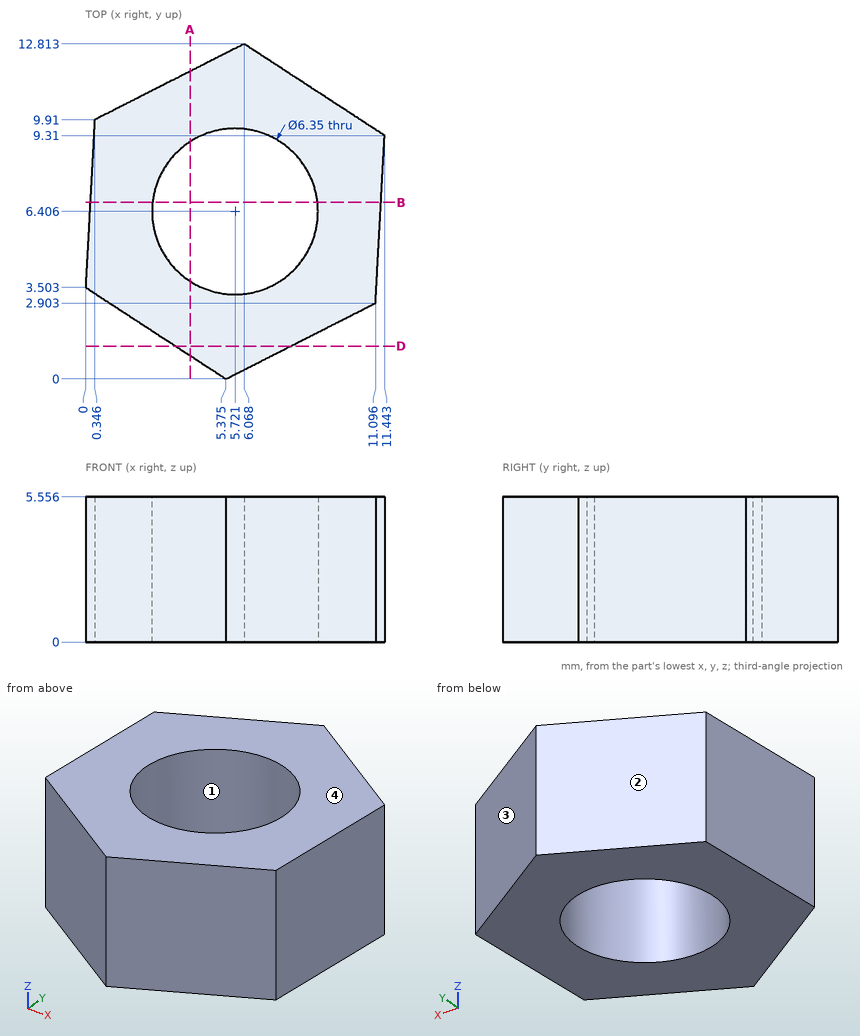
For this review, use the dimensioned drawing (mm, ordinates from the lowest corner) and the shaded views. Coordinates: 2 decimals unless noted, no trailing zeros. Write each loop counter-clockwise with the first axis right and the second up, starting at its lowest first coordinate (ties: lowest second). Pieces come first, ordered by that corner, then holes. Notation, with made-up numbers: (75.25, -31) - (89.25, -31) arc R18 ccw to (89.25, -25) - close; hole circle Ø11 at (-38, 75). An arc over 180 degrees is marked (long way). Answer in a Markdown table with one row per item. Add a question column.
Q1. Consider section A-A on x = 4. Give the boundary of the cut face in (y, z) (1 decimal).
Q2. Draft analysis for pull direction X (two halves, no side actions). For the marked faces 1, 2, 3 and 4, state which applies: +X half, -X half, draft (parallel to the pull), parting line (faces both ways), or undercut.
Q3. Consider section D-D on y = 1.25. Give the boundary of the cut face in (x, z).
Q4. Consider section B-B on y = 6.75. Give the boundary of the cut face in (x, z) (1 decimal).
Q5. Clearance check with flat-ended pins moving along their axes: pin 1 (1 mm diameter, centred on x = 7, z = 4, fed in from +Y); pin 2 (1 mm diameter, centred on x = 9.5, z = 4, fed in from +Y). State where each tip first meets the part, or that it passes through.
Q6. To check wall thickness, follow line 1 along Y through (x, z) = (6.75, 2.6); line 2 along Y through (x, z) = (4.75, 0.6) (1 decimal); line 3 along X through (y, z) = (6, 3.55) (1 decimal). State the ranges of each line that lie inside material, in increasing order. Write a range as from..to.
Answers below:
| question | item | result |
|---|---|---|
| 1 | outline | (0.9, 0) - (3.7, 0) - (3.7, 5.6) - (0.9, 5.6) - close; (9.1, 0) - (11.8, 0) - (11.8, 5.6) - (9.1, 5.6) - close |
| 2 | face 1 | undercut |
| 2 | face 2 | -X half |
| 2 | face 3 | +X half |
| 2 | face 4 | draft |
| 3 | outline | (3.46, 0) - (7.84, 0) - (7.84, 5.56) - (3.46, 5.56) - close |
| 4 | outline | (0.2, 0) - (2.6, 0) - (2.6, 5.6) - (0.2, 5.6) - close; (8.9, 0) - (11.3, 0) - (11.3, 5.6) - (8.9, 5.6) - close |
| 5 | pin 1 | y = 12.53 |
| 5 | pin 2 | y = 10.9 |
| 6 | line 1 | 0.7..3.4, 9.41..12.37 |
| 6 | line 2 | 0.4..3.4, 9.4..12.1 |
| 6 | line 3 | 0.1..2.6, 8.9..11.3 |
